```python
from build123d import *

# Parameters (mm, degrees)
SKETCH1_W               = 140
SKETCH1_H               = 140
BOSS_EXTRUDE1_DEPTH     = 140
SKETCH3_W               = 110
SKETCH3_H               = 110
CUT_EXTRUDE1_DEPTH      = 140
SKETCH4_W               = 140
SKETCH4_H               = 140
BOSS_EXTRUDE2_DEPTH     = 5
SKETCH8_W               = 8.5
SKETCH8_H               = 8.5
CUT_EXTRUDE4_DEPTH      = 140
SKETCH10_W              = 20
SKETCH10_H              = 20
CUT_EXTRUDE5_DEPTH      = 100
SKETCH12_W              = 28.647962974
SKETCH12_H              = 28.734113052
BOSS_EXTRUDE4_DEPTH     = 5
SKETCH18_W              = 23.5
SKETCH18_H              = 15
BOSS_EXTRUDE6_DEPTH     = 70
SKETCH19_W              = 15
SKETCH19_H              = 26.494211046
BOSS_EXTRUDE7_DEPTH     = 70
SKETCH24_W              = 110
SKETCH24_H              = 30
CUT_EXTRUDE8_DEPTH      = 70
CUT_EXTRUDE8_DEPTH_BACK = 70
SKETCH25_W              = 110
SKETCH25_H              = 30
CUT_EXTRUDE9_DEPTH      = 70
CUT_EXTRUDE9_DEPTH_BACK = 70
SKETCH28_W              = 4.5
SKETCH28_H              = 4.5
CUT_EXTRUDE10_DEPTH     = 66.5
SKETCH29_W              = 4.5
SKETCH29_H              = 4.5
CUT_EXTRUDE11_DEPTH     = 66.5
SKETCH30_W              = 4.5
SKETCH30_H              = 4.5
BOSS_EXTRUDE8_DEPTH     = 58
SKETCH32_W              = 4.5
SKETCH32_H              = 4.5
BOSS_EXTRUDE9_DEPTH     = 58
SKETCH34_W              = 58.042814696
SKETCH34_H              = 55
CUT_EXTRUDE20_DEPTH     = 140
SKETCH35_W              = 65.730984893
SKETCH35_H              = 63.694250149
BOSS_EXTRUDE10_DEPTH    = 5


with BuildPart() as part:
    # Sketch1 → Boss-Extrude1 (new body)
    with BuildSketch(Plane(origin=(0, 0, 0), x_dir=(1, 0, 0), z_dir=(0, 1, 0))):
        Rectangle(SKETCH1_W, SKETCH1_H)
    extrude(amount=BOSS_EXTRUDE1_DEPTH)

    # Sketch3 → Cut-Extrude1 (cut)
    with BuildSketch(Plane(origin=(0, 0, 0), x_dir=(1, 0, 0), z_dir=(0, 1, 0))):
        Rectangle(SKETCH3_W, SKETCH3_H)
    extrude(amount=CUT_EXTRUDE1_DEPTH, mode=Mode.SUBTRACT)

    # Sketch4 → Boss-Extrude2 (add)
    with BuildSketch(Plane(origin=(0, 0, 0), x_dir=(1, 0, 0), z_dir=(0, 1, 0))):
        Rectangle(SKETCH4_W, SKETCH4_H)
    extrude(amount=BOSS_EXTRUDE2_DEPTH)

    # Sketch8 → Cut-Extrude4 (cut)
    with BuildSketch(Plane(origin=(0, 0, 0), x_dir=(1, 0, 0), z_dir=(0, 1, 0))):
        with Locations((62.25, 62.25)):
            Rectangle(SKETCH8_W, SKETCH8_H)
    extrude(amount=CUT_EXTRUDE4_DEPTH, mode=Mode.SUBTRACT)

    # Sketch10 → Cut-Extrude5 (cut)
    with BuildSketch(Plane(origin=(0, 0, 0), x_dir=(1, 0, 0), z_dir=(0, 1, 0))):
        with Locations((56.5, 56.5)):
            Rectangle(SKETCH10_W, SKETCH10_H)
    extrude(amount=CUT_EXTRUDE5_DEPTH, mode=Mode.SUBTRACT)

    # Sketch12 → Boss-Extrude4 (add)
    with BuildSketch(Plane(origin=(0, 0, 0), x_dir=(1, 0, 0), z_dir=(0, 1, 0))):
        with Locations((55.676018513, 55.632943474)):
            Rectangle(SKETCH12_W, SKETCH12_H)
    extrude(amount=BOSS_EXTRUDE4_DEPTH)

    # Sketch18 → Boss-Extrude6 (add)
    with BuildSketch(Plane(origin=(0, 0, 0), x_dir=(1, 0, 0), z_dir=(0, 1, 0))):
        with Locations((58.25, 62.5)):
            Rectangle(SKETCH18_W, SKETCH18_H)
    extrude(amount=BOSS_EXTRUDE6_DEPTH)

    # Sketch19 → Boss-Extrude7 (add)
    with BuildSketch(Plane(origin=(0, 0, 0), x_dir=(1, 0, 0), z_dir=(0, 1, 0))):
        with Locations((62.5, 56.752894477)):
            Rectangle(SKETCH19_W, SKETCH19_H)
    extrude(amount=BOSS_EXTRUDE7_DEPTH)

    # Sketch24 → Cut-Extrude8 (cut, two sides)
    with BuildSketch(Plane(origin=(0, 0, 0), x_dir=(0, 0, -1), z_dir=(1, 0, 0))) as cut_extrude8_sk:
        with Locations((0, 25)):
            Rectangle(SKETCH24_W, SKETCH24_H)
    extrude(amount=CUT_EXTRUDE8_DEPTH, mode=Mode.SUBTRACT)
    extrude(cut_extrude8_sk.sketch, amount=-CUT_EXTRUDE8_DEPTH_BACK, mode=Mode.SUBTRACT)

    # Sketch25 → Cut-Extrude9 (cut, two sides)
    with BuildSketch(Plane.XY) as cut_extrude9_sk:
        with Locations((0, 25)):
            Rectangle(SKETCH25_W, SKETCH25_H)
    extrude(amount=CUT_EXTRUDE9_DEPTH, mode=Mode.SUBTRACT)
    extrude(cut_extrude9_sk.sketch, amount=-CUT_EXTRUDE9_DEPTH_BACK, mode=Mode.SUBTRACT)

    # Sketch28 → Cut-Extrude10 (cut)
    with BuildSketch(Plane.XY):
        with Locations((47.75, 137.75)):
            Rectangle(SKETCH28_W, SKETCH28_H)
    extrude(amount=-CUT_EXTRUDE10_DEPTH, mode=Mode.SUBTRACT)

    # Sketch29 → Cut-Extrude11 (cut)
    with BuildSketch(Plane(origin=(0, 0, 0), x_dir=(0, 0, -1), z_dir=(1, 0, 0))):
        with Locations((47.75, 137.75)):
            Rectangle(SKETCH29_W, SKETCH29_H)
    extrude(amount=CUT_EXTRUDE11_DEPTH, mode=Mode.SUBTRACT)

    # Sketch30 → Boss-Extrude8 (add)
    with BuildSketch(Plane.XY):
        with Locations((47.75, 137.75)):
            Rectangle(SKETCH30_W, SKETCH30_H)
    extrude(amount=-BOSS_EXTRUDE8_DEPTH)

    # Sketch32 → Boss-Extrude9 (add)
    with BuildSketch(Plane(origin=(0, 0, 0), x_dir=(0, 0, -1), z_dir=(1, 0, 0))):
        with Locations((47.75, 137.75)):
            Rectangle(SKETCH32_W, SKETCH32_H)
    extrude(amount=BOSS_EXTRUDE9_DEPTH)

    # Sketch34 → Cut-Extrude20 (cut)
    with BuildSketch(Plane(origin=(0, 0, 0), x_dir=(1, 0, 0), z_dir=(0, 1, 0))):
        with Locations((25.978592652, 27.5)):
            Rectangle(SKETCH34_W, SKETCH34_H)
    extrude(amount=CUT_EXTRUDE20_DEPTH, mode=Mode.SUBTRACT)

    # Sketch35 → Boss-Extrude10 (add)
    with BuildSketch(Plane(origin=(0, 0, 0), x_dir=(1, 0, 0), z_dir=(0, 1, 0))):
        with Locations((27.4156276, 28.86339265)):
            Rectangle(SKETCH35_W, SKETCH35_H)
    extrude(amount=BOSS_EXTRUDE10_DEPTH)


solid = part.part
```
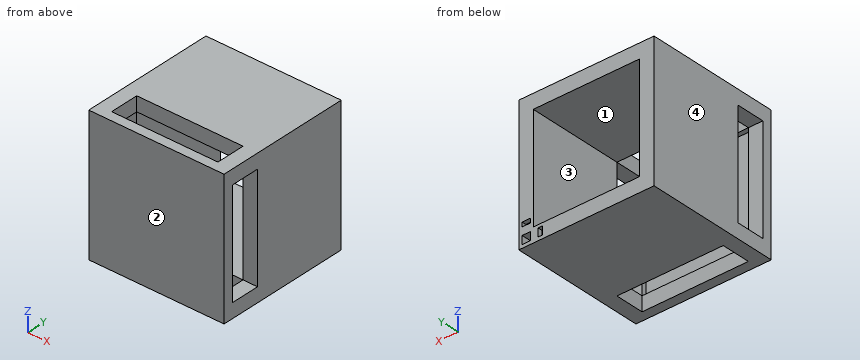
Geometry: final body of the model. Coordinates: model frame, mm. Face numbers are marked on the shaded views. Round coordinates to 2 decimals unless told otherwise and drop trailing zeros. Loops run counter-clockwise (first coordinate to the right, second up) from the corner with the lowest first, then second, coordinate; pieces in that order, holes last. Notation, with made-up numbers: (83.25, -1) -> (106.25, -1) arc R19 ccw to (106.25, 7) -> close; hole circle Ø9 at (-16, 63.25). An arc over 180 degrees is marked (long way). Use one line per item in the form item = value. Start each with the question number.
1) Section D-D on y = 125. Output: boundary loops of the cut face in (x, z).
2) Line query: L1, parallel to X at y = 83.5, z = -47; L2, parallel to X at y = 133, z = -21; L3, parallel to Y at x = -53.5, z = 60.5. Output: solid intervals per line, ascending.
3) Section B-B on y = 88. Output: boundary loops of the cut face in (x, z), then the cut area to 3 significant figures.
4) Section C-C on z = 44. Output: boundary loops of the cut face in (x, y).
5) Section A-A on x = 53. Output: boundary loops of the cut face in (y, z), then the cut area to 4 significant figures.
6) Draft query along X for the marked faces 1, 2, 3 and 4. Return one class per face: released by +X, released by -X, zero draft, split by the parting line, or undercut.
7) First-contact query: P1, Ø1, axis at x = -53, z = -7.5, coming from the +Y side. Flat tip, straight axial feed; report the tip coordinate or a pass-through.
Response:
q1.outline = (-70, -70) -> (70, -70) -> (70, 70) -> (-70, 70) -> close; hole (-55, -55) -> (55, -55) -> (55, 55) -> (-55, 55) -> close; hole (58, -66.5) -> (66.5, -66.5) -> (66.5, -58) -> (58, -58) -> close
q2.L1 = -70 to -55, 66.5 to 70
q2.L2 = -70 to -55, 55 to 70
q2.L3 = 0 to 10, 40 to 140
q3.outline = (-70, -70) -> (70, -70) -> (70, 70) -> (-70, 70) -> close; hole (-55, -55) -> (46.5, -55) -> (46.5, -66.5) -> (66.5, -66.5) -> (66.5, -46.5) -> (55, -46.5) -> (55, 55) -> (-55, 55) -> close
q3.area = 7,170 mm^2
q4.outline = (-70, 0) -> (70, 0) -> (70, 10) -> (55, 10) -> (55, 5) -> (-55, 5) -> (-55, 10) -> (-70, 10) -> close; (-70, 40) -> (-55, 40) -> (-55, 140) -> (-70, 140) -> close; (55, 40) -> (70, 40) -> (70, 140) -> (55, 140) -> close
q5.outline = (0, -70) -> (10, -70) -> (10, -55) -> (5, -55) -> (5, 55) -> (10, 55) -> (10, 70) -> (0, 70) -> close; (40, -70) -> (140, -70) -> (140, -55) -> (100, -55) -> (100, -66.5) -> (70, -66.5) -> (70, -55) -> (40, -55) -> close; (40, 55) -> (140, 55) -> (140, 70) -> (40, 70) -> close
q5.area = 3,505 mm^2
q6.face_1 = undercut
q6.face_2 = zero draft
q6.face_3 = undercut
q6.face_4 = released by -X
q7.P1 = 5
